Could you check a few things on this drawing? It's one solid part, dimensions in mm from its lowest x, y, z. A direction names the side the tool comes from. Give positions to 0.01 mm unless a question says otherwise; leave off trailing zeros. Order: outer loops, then holes, each group sorted by start corner. A loop starts at its lowest first (then second) coordinate and runs counter-clockwise, first axis right, second up.
Item 1: I'm going to push flat-ended pins straight in: pin 1 Ø4 at (y, z) = (7.5, 5) entering from -X; pin 2 Ø4 at (x, z) = (42.5, 4) entering from +Y; pin 3 Ø4 at (y, z) = (7.5, 5) entering from +X. Where does each tip first touch, or does it pass through?
Item 2: If I drill on line 1 along X through (y, z) = (1, 4); line 2 along Y through (x, z) = (9, 3.25); line 3 along X through (y, z) = (2.5, 2.5), over which ranges is the centre line in solid material (lowest first)?
Item 3: I want a section at D-D, the plane y = 15.5. Write out the boundary of the cut face in (x, z), then the cut area to 3 significant figures.
Item 4: If we mould it in two halves opening along Z, with no side actions, what happens to the marked faces 1, 2 and 3? For each: +Z half, -Z half, draft (parallel to the pull), parting line (faces both ways), or undercut.
Item 5: I want a section at C-C, the plane x = 4.75. Write out the boundary of the cut face in (y, z).
Item 6: I want a section at B-B, the plane z = 4. Write out the boundary of the cut face in (x, y).
Item 7: Which directions (+Z, -Z, +X, -X, +Y, -Y) give clear straight access to the entire face, cutting with the end or side of a thin tool? Please do the marked faces 4, 5, 6, 7 and 8.
Item 8: I want a section at A-A, the plane y = 2.5. Write out the boundary of the cut face in (x, z).
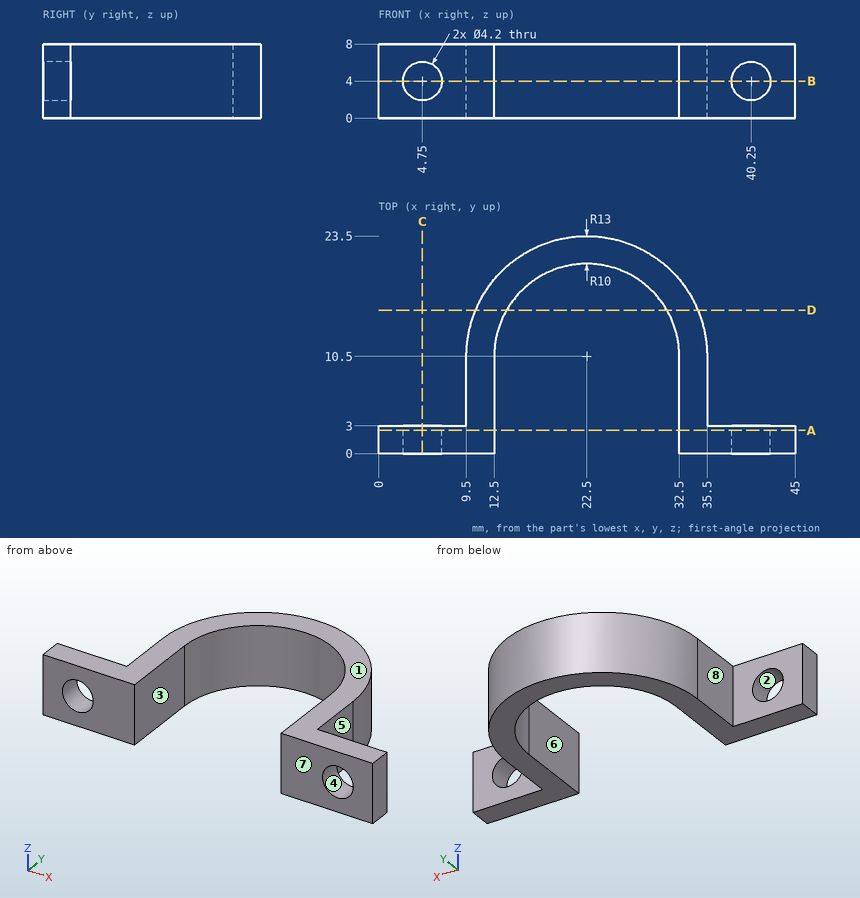
Results list:
1. pin 1: stops at x = 9.5
1. pin 2: stops at y = 3
1. pin 3: stops at x = 35.5
2. line 1: x = 0 to 2.65, 6.85 to 12.5, 32.5 to 38.15, 42.35 to 45
2. line 2: y = 0 to 3
2. line 3: x = 0 to 3.28, 6.22 to 12.5, 32.5 to 38.78, 41.72 to 45
3. outline: (10.5, 0) - (13.84, 0) - (13.84, 8) - (10.5, 8) - close; (31.16, 0) - (34.5, 0) - (34.5, 8) - (31.16, 8) - close
3. area: 53.4 mm2
4. face 1: +Z half
4. face 2: undercut
4. face 3: draft
5. outline: (0, 0) - (3, 0) - (3, 1.9) - (0, 1.9) - close; (0, 6.1) - (3, 6.1) - (3, 8) - (0, 8) - close
6. outline: (0, 0) - (2.65, 0) - (2.65, 3) - (0, 3) - close; (6.85, 0) - (12.5, 0) - (12.5, 10.5) arc R10 cw to (32.5, 10.5) - (32.5, 0) - (38.15, 0) - (38.15, 3) - (35.5, 3) - (35.5, 10.5) arc R13 ccw to (9.5, 10.5) - (9.5, 3) - (6.85, 3) - close; (42.35, 0) - (45, 0) - (45, 3) - (42.35, 3) - close
7. face 4: +Y, -Y
7. face 5: +Z, -Z, +X, +Y
7. face 6: +Z, -Z, -Y
7. face 7: +Z, -Z, +X, -X, -Y
7. face 8: +Z, -Z, -X, +Y
8. outline: (0, 0) - (12.5, 0) - (12.5, 8) - (0, 8) - close; (32.5, 0) - (45, 0) - (45, 8) - (32.5, 8) - close; hole circle Ø4.2 at (4.75, 4); hole circle Ø4.2 at (40.25, 4)
